```python
from build123d import *

# Parameters (mm, degrees)
SKETCH1_W           = 29
SKETCH1_H           = 23
BOSS_EXTRUDE1_DEPTH = 2
SKETCH2_W           = 8
SKETCH2_H           = 10
BOSS_EXTRUDE2_DEPTH = 10
CUT_EXTRUDE1_DEPTH  = 30.565013107
SKETCH5_W           = 2.5
SKETCH5_H           = 15
BOSS_EXTRUDE3_DEPTH = 3
SKETCH6_W           = 0.4
SKETCH6_H           = 0.4
BOSS_EXTRUDE4_DEPTH = 6


with BuildPart() as part:
    # Sketch1 → Boss-Extrude1 (new body)
    with BuildSketch(Plane(origin=(0, 0, 0), x_dir=(1, 0, 0), z_dir=(0, 1, 0))):
        Rectangle(SKETCH1_W, SKETCH1_H)
    extrude(amount=BOSS_EXTRUDE1_DEPTH)

    # Sketch2 → Boss-Extrude2 (add)
    with BuildSketch(Plane(origin=(0, 2, 0), x_dir=(1, 0, 0), z_dir=(0, 1, 0))):
        with Locations((10.3, -6.3)):
            Rectangle(SKETCH2_W, SKETCH2_H)
        with Locations((10.3, 6.3)):
            Rectangle(SKETCH2_W, SKETCH2_H)
    extrude(amount=BOSS_EXTRUDE2_DEPTH)

    # Sketch3 → Cut-Extrude1 (cut, through all)
    with BuildSketch(Plane.XY.offset(11.3)):
        Polygon((12.3, 12), (14.3, 12), (14.3, 8), align=None)
        Polygon((6.3, 12), (6.3, 8), (8.3, 12), align=None)
    extrude(amount=-CUT_EXTRUDE1_DEPTH, mode=Mode.SUBTRACT)

    # Sketch5 → Boss-Extrude3 (add)
    with BuildSketch(Plane(origin=(0, 2, 0), x_dir=(1, 0, 0), z_dir=(0, 1, 0))):
        with Locations((-13.15, 0)):
            Rectangle(SKETCH5_W, SKETCH5_H)
    extrude(amount=BOSS_EXTRUDE3_DEPTH)

    # Sketch6 → Boss-Extrude4 (add)
    with BuildSketch(Plane(origin=(0, 5, 0), x_dir=(1, 0, 0), z_dir=(0, 1, 0))):
        with Locations((-13.15, 6.8)):
            Rectangle(SKETCH6_W, SKETCH6_H)
        with Locations((-13.15, 4.1)):
            Rectangle(SKETCH6_W, SKETCH6_H)
        with Locations((-13.15, 1.4)):
            Rectangle(SKETCH6_W, SKETCH6_H)
        with Locations((-13.15, -1.3)):
            Rectangle(SKETCH6_W, SKETCH6_H)
        with Locations((-13.15, -4)):
            Rectangle(SKETCH6_W, SKETCH6_H)
        with Locations((-13.15, -6.7)):
            Rectangle(SKETCH6_W, SKETCH6_H)
    extrude(amount=BOSS_EXTRUDE4_DEPTH)


solid = part.part
```
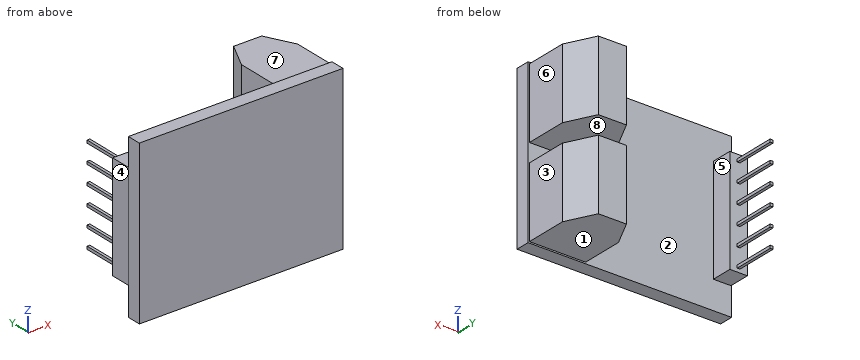
Could you check a few things on this model? Use its own coordinates, in mm. Face numbers are marked on the shaded views. A direction names the side the tool comes from. Give positions to 0.01 mm unless a question says otherwise; leave off trailing zeros. Loops run counter-clockwise (first coordinate to the right, second up) from the corner with the lowest first, then second, coordinate; pieces in that order, holes last. Notation, with made-up numbers: (70.25, -3.5) - (91.25, -3.5) arc R22 cw to (91.25, 15.5) - close; hole circle Ø5 at (66, 37). An arc over 180 degrees is marked (long way). Answer in a Markdown table with one row per item. Add a question column.
Q1. If we section it at D-D (z = -2.25): List the corners of the cut face in (x, y) for me, plus the area to 4 significant figures.
Q2. For pin 1 (1.5 mm diameter, centred on y = 7, z = 7, fed in from -X); pin 2 (1.8 mm diameter, centred on y = 4.5, z = 6.5, fed in from -X); pin 3 (4 mm diameter, centred on x = 6, y = 7.5, fed in from +Z), each with a flat end and sliding along its axis, tell me the tip position at first contact or that it passes through.
Q3. If we section it at C-C (x = 11.5): List the corners of the cut face in (y, z) for me, plus the area to 3 significant figures.
Q4. Please list where these lines run through material, in increasing order: L1, parallel to X at y = 2.5, z = 5; L2, parallel to X at y = 7.5, z = -7.25; L3, parallel to Z at x = 13.75, y = 7. Write a range as from..to.
Q5. Which directions (+Z, -Z, +X, -X, +Y, -Y) give clear straight access to the entire face, cutting with the end or side of a thin tool? Please do the marked faces 4, 5, 6, 7 and 8.
Q6. If we section it at B-B (y = 6): State how many separate pieces and enclosed holes the cut face has, plus the area to 3 significant figures.
Q7. If we section it at A-A (y = 4.25): List the corners of the cut face in (x, z) for me, plus the area to 4 significant figures.
Q8. We'd pull the mould along X, two halves only. Please class the marked faces 1, 2 and 3: +X half, -X half, draft (parallel to the pull), parting line (faces both ways), or undercut.
The answers:
| question | item | result |
|---|---|---|
| 1 | outline | (-14.5, 0) - (14.5, 0) - (14.5, 2) - (14.3, 2) - (14.3, 8) - (12.3, 12) - (8.3, 12) - (6.3, 8) - (6.3, 2) - (-11.9, 2) - (-11.9, 5) - (-14.4, 5) - (-14.4, 2) - (-14.5, 2) - close |
| 1 | area | 137.5 mm^2 |
| 2 | pin 1 | stops at x = -13.35 |
| 2 | pin 2 | stops at x = -14.4 |
| 2 | pin 3 | stops at z = 11.3 |
| 3 | outline | (0, -11.5) - (2, -11.5) - (2, -11.3) - (12, -11.3) - (12, -1.3) - (2, -1.3) - (2, 1.3) - (12, 1.3) - (12, 11.3) - (2, 11.3) - (2, 11.5) - (0, 11.5) - close |
| 3 | area | 246 mm^2 |
| 4 | L1 | x = -14.4..-11.9, 6.3..14.3 |
| 4 | L2 | x = 6.3..14.3 |
| 4 | L3 | z = -11.3..-1.3, 1.3..11.3 |
| 5 | face 4 | +Z, -Z, -X, +Y |
| 5 | face 5 | +Z, -Z, +Y |
| 5 | face 6 | +Z, -Z, +X, +Y |
| 5 | face 7 | +Z, +X, -X, +Y |
| 5 | face 8 | +X, +Y |
| 6 | separate pieces | 8 |
| 6 | enclosed holes | 0 |
| 6 | area | 161 mm^2 |
| 7 | outline | (-14.4, -7.5) - (-11.9, -7.5) - (-11.9, 7.5) - (-14.4, 7.5) - close; (6.3, -11.3) - (14.3, -11.3) - (14.3, -1.3) - (6.3, -1.3) - close; (6.3, 1.3) - (14.3, 1.3) - (14.3, 11.3) - (6.3, 11.3) - close |
| 7 | area | 197.5 mm^2 |
| 8 | face 1 | draft |
| 8 | face 2 | undercut |
| 8 | face 3 | +X half |
